Could you check a few things on this model? Use its own coordinates, in mm. A direction names the side the tool comes from. Give positions to 0.01 mm unless a question says otherwise; leave off trailing zeros. Loops run counter-clockwise (first coordinate to the right, second up) from the corner with the lowest first, then second, coordinate; pieces in that order, holes last. Notation, with made-up numbers: (61.25, 12.5) -> (69.25, 12.5) arc R27 cw to (69.25, 43.5) -> close; hole circle Ø4 at (85.5, 35). An arc over 180 degrees is marked (long way). Write item = value, one per line. Start each with the question number.
1) I want a section at D-D (z = 62). List the corners of the cut face in (x, y) for me.
2) I need wall thicknesses on probe 1 along X at (y, z) = (16, 8); probe 2 along X at (y, z) = (16, 22); probe 3 along Y at (x, z) = (18, 24.5). Which ranges of each line are inside material? Lowest first, please. Write a range as from..to.
3) On a 3-axis mill with a long thin cutter (end or side, diameter ignored), from which of +Z, -Z, +X, -X, +Y, -Y can I reach the whole of each face in a straight line? I mean faces 1 (the face through (-15.75, -24, 87)), 2 (the face through (15.62, 15.2, 13.18)), 3 (the face through (0, -26, 81)), 4 (the face through (-15.75, 23, 87)). Say none if no direction works.
4) I want a section at C-C (y = 26). List the corners of the cut face in (x, z) for me, and give its area (3 significant figures).
5) If we mould it in two halves opening along X, with no side actions, what happens to faces 5 (the face through (0, 1, 89)), 6 (the face through (15.62, -17.55, 13.18)), 7 (the face through (15.75, 23, 87))? For each: +X half, -X half, draft (parallel to the pull), parting line (faces both ways), or undercut.
6) I'm going to push flat-ended pins straight in: pin 1 Ø1.7 at (x, y) = (16.375, -16.375) entering from -Z; pin 2 Ø2 at (x, z) = (-9.5, 47.5) entering from +Y; pin 3 Ø1.6 at (y, z) = (-23.5, 88) entering from -X. Where does each tip first touch, or does it pass through?
7) I want a section at B-B (x = 6). List the corners of the cut face in (y, z) for me, and give its area (3 significant figures).
8) I want a section at A-A (z = 24). List the corners of the cut face in (x, y) for me (3 decimals).
from build123d import *

# Parameters (mm, degrees)
F0_W      = 45
F0_H      = 45
F1_DEPTH  = 89
F2_R      = 10.25
F3_DEPTH  = 25
F4_R      = 10.25
F5_DEPTH  = 27.5
F6_R      = 15.75
F7_DEPTH  = 3.5
F9_D      = 2.794
F9_DEPTH  = 26
F9_TIP    = 0.8394022848
F13_D     = 2.794
F13_DEPTH = 26
F13_TIP   = 0.8394022848
F14_D     = 2.794
F14_DEPTH = 26
F14_TIP   = 0.8394022848
F15_D     = 2.794
F15_DEPTH = 26
F15_TIP   = 0.8394022848
F16_W     = 31.5
F16_H     = 49
F17_DEPTH = 3.5
F18_R     = 8
F19_DEPTH = 8


with BuildPart() as f1:
    # F0 (on Top) → F1 (new body)
    with BuildSketch(Plane.XY):
        Rectangle(F0_W, F0_H)
    extrude(amount=F1_DEPTH)

    # F2 (on Front) → F3 (cut, symmetric)
    with BuildSketch(Plane.XZ):
        Circle(F2_R)
    extrude(amount=F3_DEPTH, both=True, mode=Mode.SUBTRACT)

    # F4 (on Right) → F5 (cut, symmetric)
    with BuildSketch(Plane.YZ):
        Circle(F4_R)
    extrude(amount=F5_DEPTH, both=True, mode=Mode.SUBTRACT)

    # F6 (on face) → F7 (join)
    with BuildSketch(Plane.XY.offset(89)):
        with Locations((0, 25)):
            Circle(F6_R)
        with Locations((0, -25)):
            Circle(F6_R)
    extrude(amount=-F7_DEPTH)

    # F9
    with Locations(Plane(origin=(0, 0, 0), x_dir=(1, 0, 0), z_dir=(0, 0, -1))):
        with Locations((16.375, 16.375)):
            Hole(F9_D / 2, depth=F9_DEPTH)
            with Locations((0, 0, -(F9_DEPTH + F9_TIP / 2))):  # 118° drill point
                Cone(0, F9_D / 2, F9_TIP, mode=Mode.SUBTRACT)

    # F13
    with Locations(Plane(origin=(0, 0, 0), x_dir=(1, 0, 0), z_dir=(0, 0, -1))):
        with Locations((16.375, -16.375)):
            Hole(F13_D / 2, depth=F13_DEPTH)
            with Locations((0, 0, -(F13_DEPTH + F13_TIP / 2))):  # 118° drill point
                Cone(0, F13_D / 2, F13_TIP, mode=Mode.SUBTRACT)

    # F14
    with Locations(Plane(origin=(0, 0, 0), x_dir=(1, 0, 0), z_dir=(0, 0, -1))):
        with Locations((-16.375, -16.375)):
            Hole(F14_D / 2, depth=F14_DEPTH)
            with Locations((0, 0, -(F14_DEPTH + F14_TIP / 2))):  # 118° drill point
                Cone(0, F14_D / 2, F14_TIP, mode=Mode.SUBTRACT)

    # F15
    with Locations(Plane(origin=(0, 0, 0), x_dir=(1, 0, 0), z_dir=(0, 0, -1))):
        with Locations((-16.375, 16.375)):
            Hole(F15_D / 2, depth=F15_DEPTH)
            with Locations((0, 0, -(F15_DEPTH + F15_TIP / 2))):  # 118° drill point
                Cone(0, F15_D / 2, F15_TIP, mode=Mode.SUBTRACT)

    # F16 (on face) → F17 (join)
    with BuildSketch(Plane.XY.offset(89)):
        Rectangle(F16_W, F16_H)
    extrude(amount=-F17_DEPTH)

    # F18 (on face) → F19 (join)
    with BuildSketch(Plane.XY.offset(89)):
        with Locations((0, 24.5)):
            Circle(F18_R)
        with Locations((0, -24.5)):
            Circle(F18_R)
    extrude(amount=-F19_DEPTH)


solid = f1.part
Answer list:
q1.outline = (-22.5, -22.5) -> (22.5, -22.5) -> (22.5, 22.5) -> (-22.5, 22.5) -> close
q2.probe_1 = -22.5..-17.72, -15.03..-6.41, 6.41..15.03, 17.72..22.5
q2.probe_2 = -22.5..-17.72, -15.03..15.03, 17.72..22.5
q2.probe_3 = -22.5..22.5
q3.face_1 = +Z, -Z, -X, -Y
q3.face_2 = -Z
q3.face_3 = -Z, +X, -X, -Y
q3.face_4 = +Z, -Z, -X, +Y
q4.outline = (-15.72, 85.5) -> (-7.86, 85.5) -> (-7.86, 81) -> (7.86, 81) -> (7.86, 85.5) -> (15.72, 85.5) -> (15.72, 89) -> (-15.72, 89) -> close
q4.area = 181 mm^2
q5.face_5 = draft
q5.face_6 = undercut
q5.face_7 = +X half
q6.pin_1 = 26.33
q6.pin_2 = 22.5
q6.pin_3 = -15.75
q7.outline = (-39.56, 85.5) -> (-29.79, 85.5) -> (-29.79, 81) -> (-22.5, 81) -> (-22.5, 8.31) -> (-6, 8.31) arc R10.25 cw to (6, 8.31) -> (22.5, 8.31) -> (22.5, 81) -> (29.79, 81) -> (29.79, 85.5) -> (39.56, 85.5) -> (39.56, 89) -> (-39.56, 89) -> close
q7.area = 3,800 mm^2
q8.outline = (-22.5, -22.5) -> (22.5, -22.5) -> (22.5, 22.5) -> (-22.5, 22.5) -> close; hole circle Ø2.794 at (-16.375, -16.375); hole circle Ø2.794 at (-16.375, 16.375); hole circle Ø2.794 at (16.375, -16.375); hole circle Ø2.794 at (16.375, 16.375)
